```python
from build123d import *

# Parameters (mm, degrees)
BOSS_EXTRUDE1_DEPTH            = 3
SKETCH2_R                      = 8.9
BOSS_EXTRUDE2_DEPTH            = 3
SKETCH3_R                      = 2
BOSS_EXTRUDE3_DEPTH            = 3
M3_CLEARANCE_HOLE1_D           = 3.4
M3_CLEARANCE_HOLE1_CSINK_D     = 3.45
M3_CLEARANCE_HOLE1_CSINK_ANGLE = 90


with BuildPart() as part:
    # Sketch1 → Boss-Extrude1 (new body)
    with BuildSketch(Plane.XY):
        with BuildLine():
            Line((-11.9, 0), (-11.9, -22.34))
            Line((-11.9, -22.34), (11.9, -22.34))
            Line((11.9, -22.34), (11.9, 0))
            ThreePointArc((11.9, 0), (0, 11.9), (-11.9, 0))
        make_face()
    extrude(amount=BOSS_EXTRUDE1_DEPTH)

    # Sketch2 → Boss-Extrude2 (add)
    with BuildSketch(Plane(origin=(0, 0, 0), x_dir=(-1, 0, 0), z_dir=(0, 0, -1))):
        Circle(SKETCH2_R)
    extrude(amount=BOSS_EXTRUDE2_DEPTH)

    # Sketch3 → Boss-Extrude3 (add)
    with BuildSketch(Plane(origin=(0, 0, -3), x_dir=(-1, 0, 0), z_dir=(0, 0, -1))):
        Circle(SKETCH3_R)
    extrude(amount=BOSS_EXTRUDE3_DEPTH)

    # M3 Clearance Hole1 (through all)
    with Locations(Plane(origin=(-5.9, -15.34, 3), x_dir=(1, 0, 0), z_dir=(0, 0, 1))):
        with Locations((0, 0), (11.8, 0)):
            CounterSinkHole(M3_CLEARANCE_HOLE1_D / 2, M3_CLEARANCE_HOLE1_CSINK_D / 2, counter_sink_angle=M3_CLEARANCE_HOLE1_CSINK_ANGLE)


solid = part.part
```
Check sheet for the modelled part. Datum: model origin and axes. Units: mm. A direction names the side the tool comes from. Give positions to 0.01 mm unless a question says otherwise; leave off trailing zeros. Write each loop counter-clockwise with the first axis right and the second up, starting at its lowest first coordinate (ties: lowest second). Pieces come first, ordered by that corner, then holes. Notation, with made-up numbers: (35, -17) - (67, -17) arc R22 cw to (67, 15) - close; hole circle Ø3 at (-28, 16.5). An arc over 180 degrees is marked (long way). Answer as a JSON object with one key per item and string values. Group by question number.
1) Release check for a two-part mould opening along X. For faces 3 (the face through (7.6, -15.3, 1.5)), 4 (the face through (0, -5, 3)), 5 (the face through (0, -2, -4)), 6 (the face through (-7.52, -14.83, 1.47)) record: pulls with the +X half, pulls with the -X half, needs draft (parallel to the pull), parting line crosses it, or undercut.
2) Sectioned sample at C-C (x = -5.9). Record the cut outline in (y, z) (3 decimals).
3) Sectioned sample at A-A (y = -15.34). Record the cut outline in (x, z) (3 decimals), then the cut area to 3 significant figures.
4) Depth check by flat-ended pin: P1, Ø4, axis at x = 5.9, y = -15.34, coming from the -Z side; P2, Ø5.5, axis at x = -2.5, y = -3, coming from the -Z side; P3, Ø3, axis at x = 4, z = -4, coming from the +Y side; P4, Ø2, axis at x = -3, z = -2.5, coming from the -Y side. Enter the tip coordinate at first touch or a pass-through.
5) Sectioned sample at B-B (z = 1.75). Record the cut outline in (x, y), then the cut area to 3 significant figures.
6) Thickness scan on probe 1 along X at (y, z) = (-15.34, 2); probe 2 along Z at (x, y) = (-5.75, -6); probe 3 along X at (y, z) = (-14, 2). Record the ranges inside material, lowest first. Write a range as from..to.
7) Access from +Z, -Z, +X, -X, +Y, -Y to the whole of each face (thin tool, end or side, straight path). Record for faces 1 (the face through (2, -9, 0)), 2 (the face through (0.262, 11.897, 1.479)).
8) Sectioned sample at D-D (x = -3). Record the cut outline in (y, z), then the cut area to 3 significant figures.
Geometry results:
{
 "1": {"face 3": "undercut", "face 4": "needs draft", "face 5": "parting line crosses it", "face 6": "undercut"},
 "2": {"outline": "(-22.34, 0) - (-17.04, 0) - (-17.04, 2.975) - (-17.065, 3) - (-22.34, 3) - close; (-13.64, 0) - (-6.663, 0) - (-6.663, -3) - (6.663, -3) - (6.663, 0) - (10.334, 0) - (10.334, 3) - (-13.615, 3) - (-13.64, 2.975) - close"},
 "3": {"outline": "(-11.9, 0) - (-7.6, 0) - (-7.6, 2.975) - (-7.625, 3) - (-11.9, 3) - close; (-4.2, 0) - (4.2, 0) - (4.2, 2.975) - (4.175, 3) - (-4.175, 3) - (-4.2, 2.975) - close; (7.6, 0) - (11.9, 0) - (11.9, 3) - (7.625, 3) - (7.6, 2.975) - close", "area": "51.0 mm^2"},
 "4": {"P1": "stops at z = 0", "P2": "stops at z = -6", "P3": "stops at y = 8.42", "P4": "stops at y = -8.67"},
 "5": {"outline": "(-11.9, -22.34) - (11.9, -22.34) - (11.9, 0) arc R11.9 ccw to (-11.9, 0) - close; hole circle Ø3.4 at (-5.9, -15.34); hole circle Ø3.4 at (5.9, -15.34)", "area": "736 mm^2"},
 "6": {"probe 1": "x = -11.9..-7.6, -4.2..4.2, 7.6..11.9", "probe 2": "z = -3..3", "probe 3": "x = -11.9..-6.95, -4.85..4.85, 6.95..11.9"},
 "7": {"face 1": "-Z", "face 2": "+Z, -Z, +Y"},
 "8": {"outline": "(-22.34, 0) - (-8.38, 0) - (-8.38, -3) - (8.38, -3) - (8.38, 0) - (11.52, 0) - (11.52, 3) - (-22.34, 3) - close", "area": "152 mm^2"}
}
